Autodesk Inventor part; units mm, degrees
ref_plane "YZ Plane" through (0, 0, 0) normal (1, 0, 0) x (0, 1, 0)
ref_plane "XZ Plane" through (0, 0, 0) normal (0, 1, 0) x (-1, 0, 0)
ref_plane "XY Plane" through (0, 0, 0) normal (0, 0, 1) x (1, 0, 0)
sketch "Sketch1" plane through (0, 0, 0) normal (0, 0, 1) x (1, 0, 0)
  circle A0 centre (0, 0) radius 10.2
  dimension "pidTechPlusDia" = 20.4
extrude "Extrusion1" add sketch "Sketch1" along normal blind 17.6
sketch "Sketch2" plane through (0, 0, 17.6) normal (0, 0, 1) x (1, 0, 0)
  circle A0 centre (0, 0) radius 10.2
  line L0 (0, 0) -> (-1.27, 0) construction
  line L1 (-1.27, 0) -> (-1.27, 4.93) construction
  line L2 (-1.27, 4.93) -> (0, 4.93) construction
  line L3 (0, 4.93) -> (0, 0) construction
  circle A1 centre (-1.27, 4.93) radius 2.415
  dimension "d3" = 1.27
  dimension "d4" = 4.93
  dimension "d5" = 4.83
extrude "Extrusion2" cut sketch "Sketch2" against normal blind 0.4 contours A1
sketch "Sketch3" plane through (0, 0, 0) normal (0, 0, -1) x (-1, 0, 0)
  circle A0 centre (0, 0) radius 10.2
  circle A1 centre (1.27, 4.93) radius 2.415
  circle A2 centre (1.27, 4.93) radius 2.415
  line L0 (0, 10.2) -> (0, -10.2) construction
  line L1 (-10.2, 0) -> (10.2, 0) construction
  circle A3 centre (4.24, 0) radius 0.785
  circle A4 centre (-3.38, 2.54) radius 0.785
  circle A5 centre (-3.38, -2.54) radius 0.785
  dimension "d8" = 4.24
  dimension "pinDia" = 1.57
  dimension "d10" = 7.62
  dimension "d11" = 5.08
extrude "Extrusion3" add sketch "Sketch3" along normal blind 4.78 contours A3 | A4 | A5
properties part number "pidtech plus"
CAD build for the part. Positions are in the model's coordinates, mm. A direction names the side the tool comes from. Coordinates: 2 decimals unless noted, no trailing zeros. Write each loop counter-clockwise with the first axis right and the second up, starting at its lowest first coordinate (ties: lowest second). Pieces come first, ordered by that corner, then holes. Notation, with made-up numbers: M 36.25,64.25 L 48.25,64.25 A25 cw 48.25,86.25 Z; hole C -28.5,2 d8. An arc over 180 degrees is marked long. Answer as a JSON object with one key per item and string values. Group by question number.
1) Tool access for faces 4 (the face through (-1.79, 2.57, 17.4)), 5 (the face through (3.96, 2.01, -2.36)), 6 (the face through (-4, 0, -4.78)): list every direction of +Z, -Z, +X, -X, +Y, -Y with a clear straight run to the whole face (end or side of a thin tool).
2) Saw through at B-B (x = -1.27). Write the cut outline in (y, z) (3 decimals), plus the area to 3 significant figures.
3) Saw through at D-D (x = 3.38). Write the cut outline in (y, z) (3 decimals).
4) Saw through at C-C (z = -1.5). Write the cut outline in (x, y) (3 decimals).
5) Mould opens along Y. For faces 1 (the face through (4, -2.06, -2.36)), 2 (the face through (3, -3, -4.78)), 3 (the face through (4.707, 9.049, 8.677)) say: +Y half, -Y half, draft (parallel to the pull), parting line (faces both ways), or undercut.
6) Saw through at A-A (y = 0). Write the cut outline in (x, z) (3 decimals).
7) Pin check, flat tips, straight feed: pin 1 Ø4.5 at (x, y) = (-1.27, 4.93) entering from +Z; pin 2 Ø1 at (x, z) = (2, 7.5) entering from +Y; pin 3 Ø12 at (x, z) = (-6.5, -1) entering from +Y. Stop position of each tip, or through.
8) Wall check: line 1 (Z direction, x = 5.5, y = 6); line 2 (Y direction, x = -1.27, z = 17.4) (3 decimals); line 3 (X direction, y = -0.25, z = 15). Give the ranges that are in metal, low to high. Write a range as from..to.
Values follow:
{
 "1": {"face 4": "+Z", "face 5": "-Z", "face 6": "-Z, +X, -X, +Y, -Y"},
 "2": {"outline": "M -10.121,0 L 10.121,0 L 10.121,17.6 L 7.345,17.6 L 7.345,17.2 L 2.515,17.2 L 2.515,17.6 L -10.121,17.6 Z", "area": "354 mm2"},
 "3": {"outline": "M -9.624,0 L -3.325,0 L -3.325,-4.78 L -1.755,-4.78 L -1.755,0 L 1.755,0 L 1.755,-4.78 L 3.325,-4.78 L 3.325,0 L 9.624,0 L 9.624,17.6 L -9.624,17.6 Z"},
 "4": {"outline": "C -4.24,0 d1.57; C 3.38,-2.54 d1.57; C 3.38,2.54 d1.57"},
 "5": {"face 1": "undercut", "face 2": "draft", "face 3": "parting line"},
 "6": {"outline": "M -10.2,0 L -5.025,0 L -5.025,-4.78 L -3.455,-4.78 L -3.455,0 L 10.2,0 L 10.2,17.6 L -10.2,17.6 Z"},
 "7": {"pin 1": "stops at z = 17.2", "pin 2": "stops at y = 10.09", "pin 3": "stops at y = 10.18"},
 "8": {"line 1": "z = 0..17.6", "line 2": "y = -10.121..2.515, 7.345..10.121", "line 3": "x = -10.2..10.2"}
}
